```python
from build123d import *

# Parameters (mm, degrees)
BOSS_EXTRUDE1_DEPTH     = 4
SKETCH2_R               = 2.75
BOSS_EXTRUDE2_DEPTH     = 50
SKETCH3_W               = 2
SKETCH3_H               = 6
CUT_EXTRUDE1_DEPTH      = 18
CUT_EXTRUDE1_DEPTH_BACK = 18
BOSS_EXTRUDE3_DEPTH     = 6
SKETCH7_R               = 2
CUT_EXTRUDE3_DEPTH      = 10
SKETCH8_R               = 2.75
BOSS_EXTRUDE4_DEPTH     = 50
SKETCH6_R               = 1.625
CUT_EXTRUDE2_DEPTH      = 13
CUT_EXTRUDE2_DEPTH_BACK = 16


with BuildPart() as part:
    # Sketch1 → Boss-Extrude1 (new body)
    with BuildSketch(Plane(origin=(0, 0, 0), x_dir=(1, 0, 0), z_dir=(0, 1, 0))):
        with BuildLine():
            Line((-15, 8), (-15, -8))
            ThreePointArc((-15, -8), (-2.516668767, -16.812685042), (12, -12.041594579))
            Line((12, -12.041594579), (12, 12.041594579))
            ThreePointArc((12, 12.041594579), (-2.516668767, 16.812685042), (-15, 8))
        make_face()
    extrude(amount=BOSS_EXTRUDE1_DEPTH)

    # Sketch2 → Boss-Extrude2 (add)
    with BuildSketch(Plane(origin=(0, 0, 0), x_dir=(1, 0, 0), z_dir=(0, 1, 0))):
        Circle(SKETCH2_R)
    extrude(amount=BOSS_EXTRUDE2_DEPTH)

    # Sketch3 → Cut-Extrude1 (cut, two sides)
    with BuildSketch(Plane.XY) as cut_extrude1_sk:
        with Locations((1.75, 12.5)):
            Rectangle(SKETCH3_W, SKETCH3_H)
    extrude(amount=CUT_EXTRUDE1_DEPTH, mode=Mode.SUBTRACT)
    extrude(cut_extrude1_sk.sketch, amount=-CUT_EXTRUDE1_DEPTH_BACK, mode=Mode.SUBTRACT)

    # Sketch4 → Boss-Extrude3 (add)
    with BuildSketch(Plane(origin=(0, 0, 0), x_dir=(1, 0, 0), z_dir=(0, 1, 0))):
        with BuildLine():
            Line((0, -7.5), (-9.5, -7.5))
            ThreePointArc((-9.5, -7.5), (-12.500612741, -6.873596088), (-15, -5.099019514))
            Line((-15, -5.099019514), (-15, 5.099019514))
            ThreePointArc((-15, 5.099019514), (-12.500612741, 6.873596088), (-9.5, 7.5))
            Line((-9.5, 7.5), (0, 7.5))
            ThreePointArc((0, 7.5), (7.5, 0), (0, -7.5))
        make_face()
    extrude(amount=BOSS_EXTRUDE3_DEPTH)

    # Sketch7 → Cut-Extrude3 (cut)
    with BuildSketch(Plane(origin=(0, 0, 0), x_dir=(1, 0, 0), z_dir=(0, 1, 0))):
        with Locations((0, 11)):
            Circle(SKETCH7_R)
        with Locations((0, -11)):
            Circle(SKETCH7_R)
    extrude(amount=CUT_EXTRUDE3_DEPTH, mode=Mode.SUBTRACT)

    # Sketch8 → Boss-Extrude4 (add)
    with BuildSketch(Plane(origin=(0, 0, 0), x_dir=(1, 0, 0), z_dir=(0, 1, 0))):
        with Locations((-9.5, 0)):
            Circle(SKETCH8_R)
    extrude(amount=BOSS_EXTRUDE4_DEPTH)

    # Sketch6 → Cut-Extrude2 (cut, two sides)
    with BuildSketch(Plane(origin=(0, 0, 0), x_dir=(0, 0, -1), z_dir=(1, 0, 0))) as cut_extrude2_sk:
        with Locations((0, 46)):
            Circle(SKETCH6_R)
    extrude(amount=CUT_EXTRUDE2_DEPTH, mode=Mode.SUBTRACT)
    extrude(cut_extrude2_sk.sketch, amount=-CUT_EXTRUDE2_DEPTH_BACK, mode=Mode.SUBTRACT)


solid = part.part
```
Geometry: final body of the model. Coordinates: model frame, mm. A direction names the side the tool comes from. Coordinates: 2 decimals unless noted, no trailing zeros. Write each loop counter-clockwise with the first axis right and the second up, starting at its lowest first coordinate (ties: lowest second). Pieces come first, ordered by that corner, then holes. Notation, with made-up numbers: M 46,55.5 L 86,55.5 A18 ccw 86,69.5 Z; hole C 68,51 d1. An arc over 180 degrees is marked long. Answer as CSV lines item,"result". Start each with the question number.
Q1. Mould query, pull axis Y, two halves, no side actions, for faces 1 (the flat face through (-10, 50, 0)), 2 (the cylindrical face through (-9.463, 46.071, 1.623)), 3 (the flat face through (-2, 0, 0)). Classes: released by +Y, released by -Y, zero draft, split by the parting line, or undercut.
Q2. Cut plane A-A on z = 0. Return the cut outline in (x, y) (3 decimals).
Q3. Reachability of faces 4 (the flat face through (-5, 5, 7.5)), 5 (the cylindrical face through (-8.23, 27.69, 2.44)), 6 (the cylindrical face through (-12.46, 4.99, 6.89)), 7 (the flat face through (2, 15.5, 0)) from +Z, -Z, +X, -X, +Y, -Y: full face, straight path, thin tool, end or side. Return the list, or none.
Q4. Line query: line 1 (Y direction, x = 0.85, z = 0) (3 decimals); line 2 (Y direction, x = -10.4, z = 0) (3 decimals); line 3 (Y direction, x = 7.5, z = 7). Output: solid intervals per line, ascending. Write a range as from..to.
Q5. Pin query (flat end, axial travel): P1, Ø10, axis at x = -2.5, y = 44.5, coming from the -Z side; P2, Ø5, axis at y = 39.5, z = -4, coming from the +X side; P3, Ø5, axis at x = -9, z = 11.5, coming from the +Y side; P4, Ø1, axis at x = -6, y = 28.5, coming from the -Z side. Return the tip coordinate at first contact, or that it passes through.
Q6. Cut plane D-D on x = -4.75. Return the cut outline in (y, z).
Q7. Cut plane B-B on y = 11. Return the cut outline in (x, z).
Q8. Cut plane C-C on z = 11. Return the cut outline in (x, y).
Findings below:
1,face 1,"released by +Y"
1,face 2,"undercut"
1,face 3,"released by -Y"
2,outline,"M -15,0 L 12,0 L 12,4 L 7.5,4 L 7.5,6 L 2.75,6 L 2.75,9.5 L 0.75,9.5 L 0.75,15.5 L 2.75,15.5 L 2.75,44.375 L -2.75,44.375 L -2.75,6 L -6.75,6 L -6.75,44.375 L -12.25,44.375 L -12.25,6 L -15,6 Z; M -12.25,47.625 L -6.75,47.625 L -6.75,50 L -12.25,50 Z; M -2.75,47.625 L 2.75,47.625 L 2.75,50 L -2.75,50 Z"
3,face 4,"+Z, +X, -X, +Y"
3,face 5,"+Y"
3,face 6,"+Z, -X, +Y"
3,face 7,"+Z, -Z, +X"
4,line 1,"y = 0..9.5, 15.5..44.375, 47.625..50"
4,line 2,"y = 0..44.375, 47.625..50"
4,line 3,"y = 0..4"
5,P1,"stops at z = -2.75"
5,P2,"stops at x = 2.3"
5,P3,"stops at y = 4"
5,P4,"passes through"
6,outline,"M 0,-16.32 L 4,-16.32 L 4,-7.5 L 6,-7.5 L 6,7.5 L 4,7.5 L 4,16.32 L 0,16.32 Z"
7,outline,"C -9.5,0 d5.5; M 0.75,-2.65 L 0.75,2.65 A2.75 ccw long Z"
8,outline,"M -12.96,0 L -2,0 L -2,4 L -12.96,4 Z; M 2,0 L 12,0 L 12,4 L 2,4 Z"
